Part model, mm, in its own coordinate system. A direction names the side the tool comes from. Round coordinates to 2 decimals unless told otherwise and drop trailing zeros. Loops run counter-clockwise (first coordinate to the right, second up) from the corner with the lowest first, then second, coordinate; pieces in that order, holes last.
(1) Cut at A-A on x = 9. List the corners of the cut face in (y, z), then the cut area to 3 significant figures.
(2) Flat gauge pins, fed straight in: pin 1 (1.5 mm diameter, centred on x = 41, z = 2.5, fed in from -Y); pin 2 (20 mm diameter, centred on x = 0, y = 0, fed in from -Z); pin 3 (2 mm diameter, centred on x = 15.5, z = 3.5, fed in from -Y). Where does each tip first touch, or does it go through?
(3) Tool access for faces 5 (the face through (-4.813, 25.357, 3.451)), 6 (the face through (48, 22.242, 3)), 7 (the face through (-46, 22.242, 3)): list every direction of +Z, -Z, +X, -X, +Y, -Y with a clear straight run to the whole face (end or side of a thin tool).
(4) Cut at B-B on z = 2.5. List the corners of the cut face in (x, y), then the cut area to 3 significant figures.
(5) Cut at C-C on y = -19. List the corners of the cut face in (x, z).
(6) Mould opens along X. For faces 1 (the face through (17.055, 15.279, 3.451)), 2 (the face through (17.83, -8.21, 3.45)), 3 (the face through (0, 12, 7)), 4 (the face through (-51.115, 15.888, 3.451)) say: +X half, -X half, draft (parallel to the pull), parting line (faces both ways), or undercut.
(7) Probe probe 1 along X at (y, z) = (19.5, 0.75); probe 2 along Y at (x, z) = (2.5, 5.75); probe 3 along Y at (x, z) = (-28, 0.75). List the from-to ranges inside material, lowest first.
(8) Cut at D-D on x = 25. List the corners of the cut face in (y, z).
from build123d import *

# Parameters (mm, degrees)
F0_R     = 11.2
F1_DEPTH = 7


with BuildPart() as f1:
    # F0 (on Top) → F1 (new body)
    with BuildSketch(Plane.XY):
        with BuildLine():
            Line((-25.988072, 22.241659), (-66.603854, 22.241659))
            ThreePointArc((-66.603854, 22.241659), (-50.942339, 15.715839), (-44.548452, 0))
            ThreePointArc((-44.548452, 0), (-17.881455, -7.399281), (0, -28.521109))
            ThreePointArc((0, -28.521109), (18.159278, -7.996654), (44.371225, 0))
            ThreePointArc((44.371225, 0), (51.493322, 15.782316), (67.558273, 22.241659))
            Line((67.558273, 22.241659), (27.147427, 22.241659))
            ThreePointArc((27.147427, 22.241659), (16.888019, 15.22177), (4.475268, 14.545086))
            Line((4.475268, 14.545086), (4.475268, 30.796813))
            Line((4.475268, 30.796813), (2.76984, 20.263286))
            ThreePointArc((2.76984, 20.263286), (-0.490537, 20.907732), (-3.750914, 20.263286))
            Line((-3.750914, 20.263286), (-5.905825, 30.596174))
            Line((-5.905825, 30.596174), (-5.905825, 14.118503))
            ThreePointArc((-5.905825, 14.118503), (-17.08841, 15.358135), (-25.988072, 22.241659))
        make_face()
        Circle(F0_R, mode=Mode.SUBTRACT)
    extrude(amount=F1_DEPTH)


solid = f1.part
Final values:
1. outline: (-15.54, 0) - (-6.67, 0) - (-6.67, 7) - (-15.54, 7) - close; (6.67, 0) - (14, 0) - (14, 7) - (6.67, 7) - close
1. area: 113 mm2
2. pin 1: stops at y = -0.26
2. pin 2: passes through
2. pin 3: stops at y = -10.59
3. face 5: +Z, -Z, +Y
3. face 6: +Z, -Z, +X, +Y
3. face 7: +Z, -Z, -X, +Y
4. outline: (-66.6, 22.24) arc R22.06 cw to (-44.55, 0) arc R47 cw to (0, -28.52) arc R50.43 cw to (44.37, 0) arc R23.21 cw to (67.56, 22.24) - (27.15, 22.24) arc R23.07 cw to (4.48, 14.55) - (4.48, 30.8) - (2.77, 20.26) arc R8.57 ccw to (-3.75, 20.26) - (-5.91, 30.6) - (-5.91, 14.12) arc R20.79 cw to (-25.99, 22.24) - close; hole circle Ø22.4 at (0, 0)
4. area: 2,250 mm2
5. outline: (-5.46, 0) - (5.98, 0) - (5.98, 7) - (-5.46, 7) - close
6. face 1: undercut
6. face 2: +X half
6. face 3: draft
6. face 4: -X half
7. probe 1: x = -55.95 to -23.55, -5.91 to 4.48, 24.43 to 56.62
7. probe 2: y = -23.95 to -10.92, 10.92 to 20.37
7. probe 3: y = -2.52 to 22.24
8. outline: (-4.31, 0) - (20.01, 0) - (20.01, 7) - (-4.31, 7) - close
